```python
from build123d import *

# Parameters (mm, degrees)
F1_DEPTH = 25.4
F3_DEPTH = 25.4
F5_DEPTH = 25.4
F6_W     = 11.27199
F6_H     = 6.35
F7_DEPTH = 25.4


with BuildPart() as f1:
    # F0 (on Front) → F1 (new body)
    with BuildSketch(Plane.XZ):
        Polygon((-19.05, 0), (0, 0), (12.7, 0), (12.7, 31.75), (-19.05, 31.75), align=None)
    extrude(amount=F1_DEPTH)

    # F2 (on face) → F3 (cut)
    with BuildSketch(Plane.XZ.offset(25.4)):
        Polygon((12.7, 0), (12.7, 31.75), (1.705643, 31.75), align=None)
    extrude(amount=-F3_DEPTH, mode=Mode.SUBTRACT)

    # F4 (on face) → F5 (cut)
    with BuildSketch(Plane.XZ.offset(25.4)):
        Polygon((-11.939476, 31.75), (-19.05, 31.75), (-19.05, 0), align=None)
    extrude(amount=-F5_DEPTH, mode=Mode.SUBTRACT)

    # F6 (on face) → F7 (cut)
    with BuildSketch(Plane.XZ.offset(25.4)):
        with Locations((-3.000005, 3.175)):
            Rectangle(F6_W, F6_H)
    extrude(amount=-F7_DEPTH, mode=Mode.SUBTRACT)


solid = f1.part
```
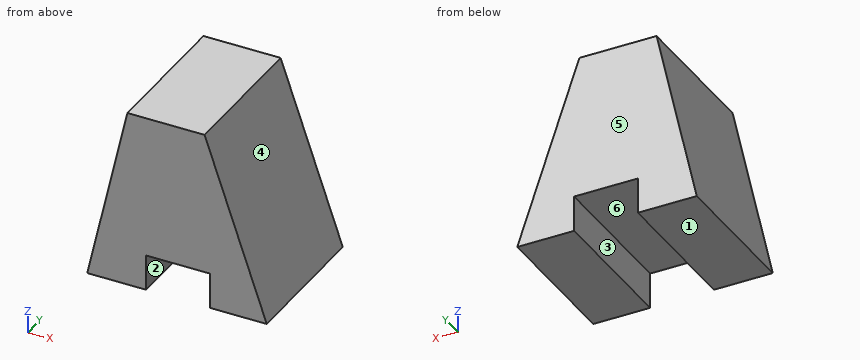
Input: part model. Units: mm. Frame: model coordinates. Face numbers are marked on the shaded views. A direction names the side the tool comes from. Give positions to 0.01 mm unless a question says otherwise; leave off trailing zeros. Order: outer loops, then holes, each group sorted by start corner. A loop starts at its lowest first (then second) coordinate and runs counter-clockwise, first axis right, second up.
1. Pin query (flat end, axial travel): pin 1 (12 mm diameter, centred on y = -10.5, z = 9.5, fed in from +X); pin 2 (1.5 mm diameter, centred on x = -2.5, y = -13, fed in from -Z); pin 3 (1.9 mm diameter, centred on y = -7, z = 3, fed in from -X); pin 4 (1 mm diameter, centred on x = 6.5, z = 21.5, fed in from -Y). Return the tip coordinate at first contact, or that it passes through.
Derived:
pin 1: stops at x = 11.49
pin 2: stops at z = 6.35
pin 3: stops at x = -18.59
pin 4: passes through
2. Section C-C on x = 0.5. Return the cut outline in (y, z), and give its area (3 significant figures).
Derived:
outline: (-25.4, 6.35) - (0, 6.35) - (0, 31.75) - (-25.4, 31.75) - close
area: 645 mm2
3. Section B-B on z = 2. Return the cut outline in (x, y), and give its area (3 significant figures).
Derived:
outline: (-18.6, -25.4) - (-8.64, -25.4) - (-8.64, 0) - (-18.6, 0) - close; (2.64, -25.4) - (12.01, -25.4) - (12.01, 0) - (2.64, 0) - close
area: 491 mm2
4. Reachability of the marked faces 1 and 2 from +Z, -Z, +X, -X, +Y, -Y: full face, straight path, thin tool, end or side. Return the list, or none.
Derived:
face 1: -Z, +X, -X, +Y, -Y
face 2: -Z, +Y, -Y
5. Section D-D on z = 13.5. Return the cut outline in (x, y).
Derived:
outline: (-16.03, -25.4) - (8.03, -25.4) - (8.03, 0) - (-16.03, 0) - close
6. Material intervals for L1, parallel to Z at x = -3.5, y = -18; L2, parallel to X at y = -2, z = 1.5; L3, parallel to X at y = -8, z = 19, sorted ascending.
Derived:
L1: z = 6.35 to 31.75
L2: x = -18.71 to -8.64, 2.64 to 12.18
L3: x = -14.79 to 6.12
7. Section A-A on y = -23.5. Return the cut outline in (x, z), and give its area (3 significant figures).
Derived:
outline: (-19.05, 0) - (-8.64, 0) - (-8.64, 6.35) - (2.64, 6.35) - (2.64, 0) - (12.7, 0) - (1.71, 31.75) - (-11.94, 31.75) - close
area: 649 mm2
8. Mould query, pull axis X, two halves, no side actions, for the marked faces 3, 4, 5 and 6. Classes: released by +X, released by -X, zero draft, split by the parting line, or undercut.
Derived:
face 3: undercut
face 4: released by +X
face 5: zero draft
face 6: undercut
